Print and shaded views of the part. All mm, measured from the part's lowest x, y and z. A direction names the side the tool comes from. Round coordinates to 2 decimals unless told otherwise and drop trailing zeros. Order: outer loops, then holes, each group sorted by start corner. A loop starts at its lowest first (then second) coordinate and runs counter-clockwise, first axis right, second up. Notation, with made-up numbers: (32.5, -33.75) - (46.5, -33.75) arc R31 ccw to (46.5, -0.75) - close; hole circle Ø2 at (40.5, 20). An arc over 180 degrees is marked (long way). Return JSON: item names as keys, results as strings. Group by question number.
Item 1: Saw through at C-C on x = 43.4. List the corners of the cut face in (y, z), and give its area (3 significant figures).
Item 2: Saw through at A-A on x = 9. List the corners of the cut face in (y, z), and give its area (3 significant figures).
Item 3: Drop flat-ended pins along their axis: pin 1 (4 mm diameter, centred on x = 44.5, y = 7, fed in from +Z); pin 2 (3 mm diameter, centred on x = 12, y = 27.5, fed in from +Z). Give the stop position or say it passes through.
Item 4: Tool access for the marked faces 1, 2 and 3: list every direction of +Z, -Z, +X, -X, +Y, -Y with a clear straight run to the whole face (end or side of a thin tool).
Item 5: Two-plate mould, pull along Y, no slides. Class the marked faces 4, 5, 6 and 7: released by +Y, released by -Y, zero draft, split by the parting line, or undercut.
Item 6: Saw through at D-D on y = 28. List the corners of the cut face in (x, z), and give its area (3 significant figures).
Item 7: Saw through at B-B on y = 21.5. List the corners of the cut face in (x, z).
Item 8: Probe probe 1 along X at (y, z) = (20, 5); probe 2 along Z at (x, y) = (27.5, 2.5); probe 3 along X at (y, z) = (34.5, 28). List the from-to ranges inside material, lowest first.
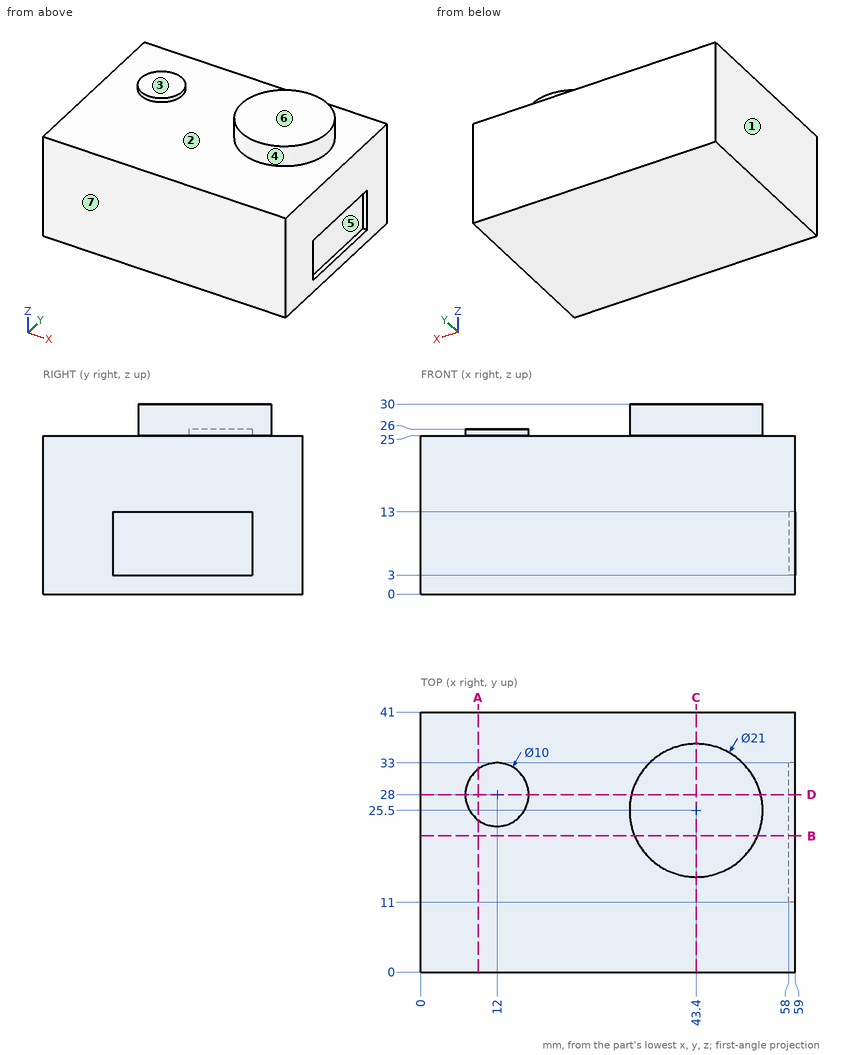
Filled in:
{
 "1": {"outline": "(0, 0) - (41, 0) - (41, 25) - (36, 25) - (36, 30) - (15, 30) - (15, 25) - (0, 25) - close", "area": "1,130 mm^2"},
 "2": {"outline": "(0, 0) - (41, 0) - (41, 25) - (32, 25) - (32, 26) - (24, 26) - (24, 25) - (0, 25) - close", "area": "1,030 mm^2"},
 "3": {"pin 1": "stops at z = 25", "pin 2": "stops at z = 26"},
 "4": {"face 1": "+Z, -Z, -X, +Y, -Y", "face 2": "+Z", "face 3": "+Z, -X, +Y, -Y"},
 "5": {"face 4": "split by the parting line", "face 5": "undercut", "face 6": "zero draft", "face 7": "released by -Y"},
 "6": {"outline": "(0, 0) - (59, 0) - (59, 3) - (58, 3) - (58, 13) - (59, 13) - (59, 25) - (53.6, 25) - (53.6, 30) - (33.2, 30) - (33.2, 25) - (17, 25) - (17, 26) - (7, 26) - (7, 25) - (0, 25) - close", "area": "1,580 mm^2"},
 "7": {"outline": "(0, 0) - (59, 0) - (59, 3) - (58, 3) - (58, 13) - (59, 13) - (59, 25) - (53.11, 25) - (53.11, 30) - (33.69, 30) - (33.69, 25) - (0, 25) - close"},
 "8": {"probe 1": "x = 0 to 58", "probe 2": "z = 0 to 25", "probe 3": "x = 37.99 to 48.81"}
}
